Geometry: final body of the model. Coordinates: model frame, mm. A direction names the side the tool comes from. Round coordinates to 2 decimals unless told otherwise and drop trailing zeros. Write each loop counter-clockwise with the first axis right and the second up, starting at its lowest first coordinate (ties: lowest second). Pieces come first, ordered by that corner, then holes. Notation, with made-up numbers: (53.5, -20) -> (86.5, -20) arc R23 ccw to (86.5, 17) -> close; hole circle Ø7 at (80.25, 24). An arc over 180 degrees is marked (long way). Use one line per item in the form item = value. Start each with the question number.
1. Reachability of faces 1 (the face through (-2.17, -6.23, -9.76)), 2 (the face through (0, -20, 0)), 3 (the face through (-0.1, 0, 10.2)) from +Z, -Z, +X, -X, +Y, -Y: full face, straight path, thin tool, end or side. Return the list, or none.
2. Cut plane D-D, the plane y = -2. Return the cut outline in (x, z), plus the area to 3 significant figures.
3. Pin query (flat end, axial travel): pin 1 Ø10 at (y, z) = (-5, 5.5) entering from +X; pin 2 Ø12 at (y, z) = (-10.5, -2) entering from -X; pin 3 Ø2 at (x, y) = (-3.5, -7.5) entering from +Z. Return the tip coordinate at first contact, or that it passes through.
4. Cut plane C-C, the plane y = -9.5. Return the cut outline in (x, z).
5. Draft query along Z for faces 4 (the face through (0, 0, 0)), 5 (the face through (4, 2.5, 7)), 6 (the face through (-7.493, -13.662, 0.33)). Return one class per face: pulls with the +Z half, pulls with the -Z half, needs draft (parallel to the pull), parting line crosses it, or undercut.
6. Line query: L1, parallel to Z at x = 0, y = 0.75; L2, parallel to Y at x = -3.25, z = -4; L3, parallel to Y at x = -6.5, z = 6.5. Output: solid intervals per line, ascending.
```python
from build123d import *

# Parameters (mm, degrees)
F0_R        = 10
F0_R_2      = 7.5
F1_DEPTH    = 2.5
F1_FACE_R   = 10
F1_FACE_R_2 = 7.5
F2_R        = 12.5
F2_R_2      = 10
F3_DEPTH    = 5
F4_R        = 10
F4_R_2      = 7.5
F5_DEPTH    = 2.5
F7_SIZE     = 2.49999
F8_R        = 5
F6_R        = 7.5
F9_DEPTH    = 20


# Not quite as in the source:
# - a fillet or chamfer is up to 0.001 mm smaller than in the source, because OpenCascade refuses the exact size


with BuildPart() as f1:
    # F0 (on Front) → F1 (new body)
    with BuildSketch(Plane.XZ):
        Circle(F0_R)
        Circle(F0_R_2, mode=Mode.SUBTRACT)
    extrude(amount=F1_DEPTH)

    # F1_face (on face) + F2 (on Front) → F3 (join)
    with BuildSketch(Plane.XZ.offset(2.5)):
        Circle(F1_FACE_R)
        Circle(F1_FACE_R_2, mode=Mode.SUBTRACT)
    with BuildSketch(Plane.XZ):
        Circle(F2_R)
        Circle(F2_R_2, mode=Mode.SUBTRACT)
    extrude(amount=F3_DEPTH)

    # F4 (on Front) → F5 (join)
    with BuildSketch(Plane.XZ):
        Circle(F4_R)
        Circle(F4_R_2, mode=Mode.SUBTRACT)
    extrude(amount=-F5_DEPTH)

    # F7 (size 2.5 in the source; OpenCascade refuses exactly that, so slightly less here)
    f7_edges = [f1.edges().sort_by_distance(p)[0] for p in [
        (-12.5, -5, 0),
    ]]
    chamfer(f7_edges, length=F7_SIZE)

    # F8 (on Front) + F6 (on Front) → F9 (join)
    with BuildSketch(Plane.XZ):
        Circle(F8_R)
    with BuildSketch(Plane.XZ):
        Circle(F6_R)
    extrude(amount=F9_DEPTH)


solid = f1.part
```
Outcome:
q1.face_1 = -Y
q1.face_2 = +Z, -Z, +X, -X, -Y
q1.face_3 = +Y
q2.outline = circle Ø25 at (0, 0)
q2.area = 491 mm^2
q3.pin_1 = 12.45
q3.pin_2 = -10.38
q3.pin_3 = 9.68
q4.outline = circle Ø15 at (0, 0)
q5.face_4 = undercut
q5.face_5 = needs draft
q5.face_6 = parting line crosses it
q6.L1 = -10 to -7.5, 7.5 to 10
q6.L2 = -20 to 0
q6.L3 = -7.5 to 2.5
